Work out the finished part from the listing and answer in its coordinate system (mm). A direction names the side the tool comes from. Give positions to 0.01 mm unless a question says otherwise; leave off trailing zeros. Order: outer loops, then holes, each group sorted by start corner. A loop starts at its lowest first (then second) coordinate and runs counter-clockwise, first axis right, second up. Notation, with made-up numbers: (47, 67.5) -> (91, 67.5) arc R10 cw to (91, 82.5) -> close; hole circle Ø9 at (80.25, 46). An arc over 180 degrees is marked (long way). Use a Markdown table: item, result. Add a question column.
```python
from build123d import *

# Parameters (mm, degrees)
F0_W     = 63.5
F0_H     = 114.3
F1_DEPTH = 25.4
F3_D     = 5.1054
F3_DEPTH = 22.86
F3_TIP   = 1.5338169022
F5_DEPTH = 25.4
F6_R     = 6.746875
F7_DEPTH = 30.1625
F9_D     = 11.50874


with BuildPart() as f1:
    # F0 (on Top) → F1 (new body)
    with BuildSketch(Plane.XY):
        with Locations((31.75, -57.15)):
            Rectangle(F0_W, F0_H)
    extrude(amount=F1_DEPTH)

    # F3
    with Locations(Plane(origin=(0, 0, 0), x_dir=(-1, 0, 0), z_dir=(0, 1, 0))):
        with Locations((-57.15, 12.7), (-6.35, 12.7)):
            Hole(F3_D / 2, depth=F3_DEPTH)
            with Locations((0, 0, -(F3_DEPTH + F3_TIP / 2))):  # 118° drill point
                Cone(0, F3_D / 2, F3_TIP, mode=Mode.SUBTRACT)

    # F4 (on face) → F5 (cut, through all)
    with BuildSketch(Plane.XY.offset(25.4)):
        with BuildLine():
            Line((33.3375, -114.3), (33.3375, -84.9413116145))
            ThreePointArc((33.3375, -84.9413116145), (31.75, -42), (30.1625, -84.9413116145))
            Line((30.1625, -84.9413116145), (30.1625, -114.3))
            Line((30.1625, -114.3), (33.3375, -114.3))
        make_face()
    extrude(amount=-F5_DEPTH, mode=Mode.SUBTRACT)

    # F6 (on face) → F7 (cut, through all)
    with BuildSketch(Plane.YZ.offset(63.5)):
        with Locations((-95.25, 12.7)):
            Circle(F6_R)
    extrude(amount=-F7_DEPTH, mode=Mode.SUBTRACT)

    # F9 (through all)
    with Locations(Plane.YZ.offset(30.1625)):
        with Locations((-95.25, 12.7)):
            Hole(F9_D / 2)


solid = f1.part
```
1) Which of the six approach directions +Z, -Z, +X, -X, +Y, -Y give full straight-line access (tool end or side, diameter ignored) to faces 1 (the cylindrical face through (5.797, -11.59, 10.208)), 2 (the cylindrical face through (48.63, -88.815, 14.727)), 3 (the flat face through (17, -44, 25.4)), 4 (the flat face through (33.338, -103, 13))?
2) The part is cut by section C-C, the plane y = -95.25. Determine the outline of the cut face in (x, z), then the cut area to 3 significant figures.
3) Determine the mould class of faces 5 (the flat face through (63.5, -58, 13)), 6 (the cylindrical face through (14.87, -89.5, 12.95)), 7 (the cylindrical face through (54.6, -11.6, 12.8)), 8 (the cylindrical face through (32.67, -42.02, 12.88)) for opening direction X: released by +X, released by -X, zero draft, split by the parting line, or undercut.
4) Straight lines are drawn through the part: line 1 (Z direction, x = 57, y = -14); line 2 (X direction, y = -4.75, z = 12.7); line 3 (X direction, y = -88, z = 12). For each, find the intervals that lie inside material, in ascending order.
5) The part is cut by section B-B, the plane x = 26.5. Determine the outline of the cut face in (y, z).
6) The part is cut by section D-D, the plane z = 3. Determine the outline of the cut face in (x, y).
7) A flat-ended cylindrical pin translates along its axis: pin 1 (4.5 mm diameter, centred on x = 57.15, z = 12.7, fed in from +Y). Find the tip coordinate at first contact, or state that the pin passes through.
8) The part is cut by section A-A, the plane y = -63.5. Determine the outline of the cut face in (x, z).
A:
| question | item | result |
|---|---|---|
| 1 | face 1 | +Y |
| 1 | face 2 | +X |
| 1 | face 3 | +Z, +X, -X, +Y, -Y |
| 1 | face 4 | +Z, -Z, -Y |
| 2 | outline | (0, 0) -> (30.16, 0) -> (30.16, 6.95) -> (0, 6.95) -> close; (0, 18.45) -> (30.16, 18.45) -> (30.16, 25.4) -> (0, 25.4) -> close; (33.34, 0) -> (63.5, 0) -> (63.5, 5.95) -> (33.34, 5.95) -> close; (33.34, 19.45) -> (63.5, 19.45) -> (63.5, 25.4) -> (33.34, 25.4) -> close |
| 2 | area | 778 mm^2 |
| 3 | face 5 | released by +X |
| 3 | face 6 | zero draft |
| 3 | face 7 | undercut |
| 3 | face 8 | undercut |
| 4 | line 1 | 0 to 10.15, 15.25 to 25.4 |
| 4 | line 2 | 0 to 3.8, 8.9 to 54.6, 59.7 to 63.5 |
| 4 | line 3 | 0 to 30.16, 33.34 to 63.5 |
| 5 | outline | (-114.3, 0) -> (-84.35, 0) -> (-84.35, 25.4) -> (-114.3, 25.4) -> close; (-42.65, 0) -> (0, 0) -> (0, 25.4) -> (-42.65, 25.4) -> close; hole circle Ø11.51 at (-95.25, 12.7) |
| 6 | outline | (0, -114.3) -> (30.16, -114.3) -> (30.16, -84.94) arc R21.5 cw (long way) to (33.34, -84.94) -> (33.34, -114.3) -> (63.5, -114.3) -> (63.5, 0) -> (0, 0) -> close |
| 7 | pin 1 | y = -23.04 |
| 8 | outline | (0, 0) -> (10.25, 0) -> (10.25, 25.4) -> (0, 25.4) -> close; (53.25, 0) -> (63.5, 0) -> (63.5, 25.4) -> (53.25, 25.4) -> close |
